from build123d import *

# Parameters (mm, degrees)
SKETCH_1_R          = 5.25
EXTRUDE_1_DEPTH     = 130
SKETCH_2_R          = 6
EXTRUDE_2_DEPTH     = 42
SKETCH_3_R          = 7
EXTRUDE_3_DEPTH     = 3
SKETCH_4_R          = 6
EXTRUDE_4_DEPTH     = 12
SKETCH_5_R          = 4.5
EXTRUDE_5_DEPTH     = 8
EXTRUDE_START       = 8
SKETCH_6_R          = 4.5
EXTRUDE_6_DEPTH     = 8
CUT_EXTRUDE_1_DEPTH = 10
FILLET_2_R          = 0.2
FILLET_4_R          = 0.2
FILLET_5_R          = 0.2
SKETCH_19_R         = 4.5
EXTRUDE_7_DEPTH     = 12
FILLET_6_R          = 0.2
FILLET_7_R          = 0.2
CHAMFER_1_SIZE      = 0.5


with BuildPart() as part:
    # Эскиз1 → Бобышка-Вытянуть1 (new body)
    with BuildSketch(Plane.XY):
        Circle(SKETCH_1_R)
    extrude(amount=EXTRUDE_1_DEPTH)

    # Эскиз2 → Бобышка-Вытянуть2 (add)
    with BuildSketch(Plane.XY.offset(130)):
        with Locations(Location((0, 0, 0), (0, 0, 180))):
            Circle(SKETCH_2_R)
    extrude(amount=EXTRUDE_2_DEPTH)

    # Эскиз3 → Бобышка-Вытянуть3 (add)
    with BuildSketch(Plane.XY.offset(172)):
        Circle(SKETCH_3_R)
    extrude(amount=EXTRUDE_3_DEPTH)

    # Эскиз4 → Бобышка-Вытянуть4 (add)
    with BuildSketch(Plane.XY.offset(175)):
        with Locations(Location((0, 0, 0), (0, 0, 180))):
            Circle(SKETCH_4_R)
    extrude(amount=EXTRUDE_4_DEPTH)

    # Эскиз5 → Бобышка-Вытянуть5 (add)
    with BuildSketch(Plane.XY.offset(187)):
        Circle(SKETCH_5_R)
    extrude(amount=EXTRUDE_5_DEPTH)

    # Эскиз6 → Бобышка-Вытянуть6 (add)
    with BuildSketch(Plane(origin=(0, 0, 0), x_dir=(-1, 0, 0), z_dir=(0, 0, -1)).offset(EXTRUDE_START)):
        with Locations(Location((0, 0, 0), (0, 0, 180))):
            Circle(SKETCH_6_R)
    extrude(amount=-EXTRUDE_6_DEPTH)

    # Эскиз18 → Вырез-Вытянуть1 (cut)
    with BuildSketch(Plane(origin=(0, 12, 0), x_dir=(1, 0, 0), z_dir=(0, 1, 0))):
        with BuildLine():
            Line((-2, -160.373495066), (-2, -152.373495066))
            ThreePointArc((-2, -152.373495066), (0, -150.373495066), (2, -152.373495066))
            Line((2, -152.373495066), (2, -160.373495066))
            ThreePointArc((2, -160.373495066), (0, -162.373495066), (-2, -160.373495066))
        make_face()
    extrude(amount=-CUT_EXTRUDE_1_DEPTH, mode=Mode.SUBTRACT)

    # Скругление2
    fillet_2_edges = [part.edges().sort_by_distance(p)[0] for p in [
        (-4.5, 0, 0),
    ]]
    fillet(fillet_2_edges, radius=FILLET_2_R)

    # Скругление4
    fillet_4_edges = [part.edges().sort_by_distance(p)[0] for p in [
        (6, 0, 175),
    ]]
    fillet(fillet_4_edges, radius=FILLET_4_R)

    # Скругление5
    fillet_5_edges = [part.edges().sort_by_distance(p)[0] for p in [
        (-4.5, 0, 187),
    ]]
    fillet(fillet_5_edges, radius=FILLET_5_R)

    # Эскиз19 → Бобышка-Вытянуть7 (add)
    with BuildSketch(Plane.XY.offset(195)):
        Circle(SKETCH_19_R)
    extrude(amount=EXTRUDE_7_DEPTH)

    # Скругление6
    fillet_6_edges = [part.edges().sort_by_distance(p)[0] for p in [
        (-5.25, 0, 130),
    ]]
    fillet(fillet_6_edges, radius=FILLET_6_R)

    # Скругление7
    fillet_7_edges = [part.edges().sort_by_distance(p)[0] for p in [
        (6, 0, 172),
    ]]
    fillet(fillet_7_edges, radius=FILLET_7_R)

    # Фаска1
    chamfer_1_edges = [part.edges().sort_by_distance(p)[0] for p in [
        (-4.5, 0, -8),
        (-4.5, 0, 207),
    ]]
    chamfer(chamfer_1_edges, length=CHAMFER_1_SIZE)


solid = part.part
The model under review builds one solid part; all positions refer to its coordinate system, in mm. A direction names the side the tool comes from. Round coordinates to 2 decimals unless told otherwise and drop trailing zeros. Order: outer loops, then holes, each group sorted by start corner. A loop starts at its lowest first (then second) coordinate and runs counter-clockwise, first axis right, second up. Notation, with made-up numbers: (40.5, 71.5) -> (99.5, 71.5) arc R5 ccw to (99.5, 77.5) -> close; hole circle Ø4 at (-38.5, 52). An arc over 180 degrees is marked (long way). Return JSON: item names as keys, results as strings.
1. Insertion check: P1, Ø4.5, axis at x = -1, z = 158, coming from the +Y side; P2, Ø4, axis at y = 4, z = 157.5, coming from the -X side; P3, Ø2, axis at x = 4, y = -5, coming from the +Z side. Each pin has a flat end and moves straight along its axis. Give the tip position at first contact, or say it passes through.
Answer block:
{"P1": "stops at y = 5.66", "P2": "stops at x = -5.66", "P3": "stops at z = 187"}
2. For L1, parallel to X at y = 4.5, z = 160; L2, parallel to X at y = 2.75, z = 30.5; L3, parallel to X at y = 4.5, z = 170, list the stretches that pass through material, from the lowest coordinate up. Write a range as [from, to].
Answer block:
{"L1": "x = [-3.97, -2], [2, 3.97]", "L2": "x = [-4.47, 4.47]", "L3": "x = [-3.97, 3.97]"}
3. For faces 5 (the face through (6.466, -2.681, 173.479)), 6 (the face through (-4, -3, 0)), 7 (the face through (0, 2, 156)), 8 (the face through (4, 3, 187)), list the 3-axis set-ups (+Z, -Z, +X, -X, +Y, -Y) from which the entire face can be reached by the end or side of a thin tool; tool diameter is ignored.
Answer block:
{"face 5": "+Z, -Z", "face 6": "-Z", "face 7": "+Y", "face 8": "+Z"}
4. Take a section at A-A (z = 110). Write out the cut boundary in (x, y), then the cut area to 3 significant figures.
Answer block:
{"outline": "circle Ø10.5 at (0, 0)", "area": "86.6 mm²"}
5. The part is to be moulded in two halves that separate along Z. For faces 1 (the face through (-0.044, 4.03, 150.374)), 2 (the face through (-2, 4, 156)), 3 (the face through (-5.723, -1.802, 181.017)), 4 (the face through (-4, -5, 175)), say which applies: +Z half, -Z half, draft (parallel to the pull), parting line (faces both ways), or undercut.
Answer block:
{"face 1": "undercut", "face 2": "undercut", "face 3": "draft", "face 4": "+Z half"}
